Autodesk Inventor part; units mm, degrees
ref_plane "YZ Plane" through (0, 0, 0) normal (1, 0, 0) x (0, 1, 0)
ref_plane "XZ Plane" through (0, 0, 0) normal (0, 1, 0) x (-1, 0, 0)
ref_plane "XY Plane" through (0, 0, 0) normal (0, 0, 1) x (1, 0, 0)
sketch "Sketch1" plane through (0, 0, 0) normal (0, 1, 0) x (-1, 0, 0)
  line L0 (-414.3, 17.5) -> (-414.3, 107.5) construction
  line L1 (-417.5, -14.3) -> (417.5, -14.3) construction
  line L2 (417.5, 139.3) -> (-417.5, 139.3) construction
  line L3 (414.3, 107.5) -> (414.3, 17.5) construction
  line L4 (417.5, 110.7) -> (-417.5, 110.7) construction
  circle A0 centre (-400, 0) radius 2 construction
  circle A1 centre (-400, 125) radius 2 construction
  circle A2 centre (400, 0) radius 2 construction
  circle A3 centre (400, 125) radius 2 construction
  circle A4 centre (0, 125) radius 2 construction
  circle A5 centre (0, 0) radius 2 construction
  arc A6 (-255.8176, 91.7662) -> (-287.0162, 60.5676) centre (-251.75, 56.5) ccw construction
  arc A7 (-247.75, 95.5) -> (-255.75, 95.5) centre (-251.75, 95.5) ccw construction
  arc A8 (255.75, 95.5) -> (247.75, 95.5) centre (251.75, 95.5) ccw construction
  line L5 (417.5, 14.3) -> (-417.5, 14.3) construction
  line L6 (0, -14.3) -> (0, 139.3) construction
  line L7 (-414.3, 139.3) -> (414.3, 139.3)
  line L8 (414.3, 139.3) -> (414.3, -14.3)
  line L9 (-414.3, -14.3) -> (-414.3, 139.3)
  line L10 (-414.3, 139.3) -> (414.3, -14.3) construction
  line L11 (414.3, 139.3) -> (-414.3, -14.3) construction
  line L12 (-251.75, 99.5) -> (-251.75, 14.3) construction
  line L13 (251.75, 99.5) -> (251.75, 14.3) construction
  line L14 (-294.75, 56.5) -> (-294.75, -14.3)
  line L15 (-208.75, 56.5) -> (-208.75, -14.3)
  line L16 (209.15, 56.9) -> (209.15, -14.3)
  line L17 (294.35, 56.9) -> (294.35, -14.3)
  arc A9 (-260.011, 14.301) -> (-260.0059, 14.3) centre (-251.75, 56.5) ccw
  arc A10 (-208.75, 56.5) -> (-294.75, 56.5) centre (-251.75, 56.5) ccw
  arc A11 (294.35, 56.9) -> (209.15, 56.9) centre (251.75, 56.9) ccw
  line L18 (-294.75, -14.3) -> (-414.3, -14.3)
  line L19 (414.3, -14.3) -> (294.35, -14.3)
  line L20 (209.15, -14.3) -> (-208.75, -14.3)
  circle A12 centre (-400, 0) radius 3
  circle A13 centre (-400, 125) radius 3
  circle A14 centre (0, 0) radius 3
  circle A15 centre (0, 125) radius 3
  circle A16 centre (400, 125) radius 3
  circle A17 centre (400, 0) radius 3
  point P0 (0, 0)
  point P1 (0, 62.5)
  dimension "d0" = 828.6
  dimension "d1" = 43
  dimension "d2" = 125
  dimension "d3" = 1
  dimension "d4" = 1
  dimension "d5" = 1
  dimension "d6" = 1
  dimension "d7" = 1
  dimension "d8" = 1
extrude "Extrusion1" add sketch "Sketch1" along normal mid plane 2
fillet "Fillet1" radius 2 8 edges at (414.3, 0, -14.3) (208.75, 0, -14.3) (294.75, 0, -14.3) (-209.15, 0, -14.3) (-294.35, 0, -14.3) (-414.3, 0, -14.3) (414.3, 0, 139.3) (-414.3, 0, 139.3)
properties part number "Cover_LeftRight" material "Steel, Galvanized"
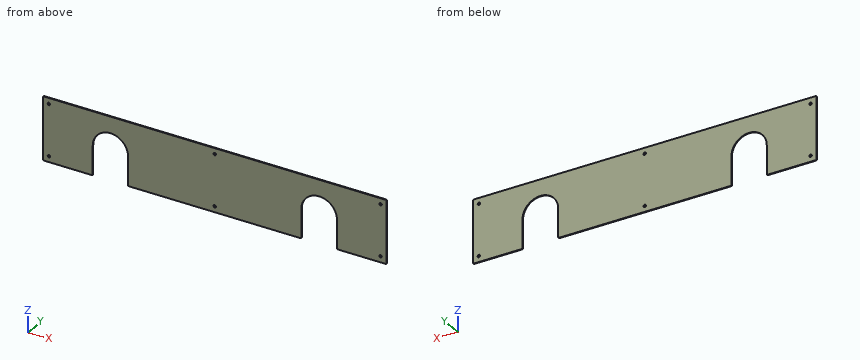
Read the model definition and answer for the solid it produces. Units are mm, in the model's axes. Coordinates: 2 decimals unless noted, no trailing zeros. Write each loop counter-clockwise with the first axis right and the second up, starting at its lowest first coordinate (ties: lowest second). Pieces come first, ordered by that corner, then holes. Notation, with made-up numbers: M 61,68.25 L 94,68.25 A12 ccw 94,81.25 Z; hole C 30,28 d5. An arc over 180 degrees is marked long. Use a Markdown table: item, result.
Q1. The part is cut by section D-D, the plane z = 81. Write down the section's boundary in (x, y).
Answer block:
| item | result |
|---|---|
| outline | M -414.3,-1 L -286.88,-1 L -286.88,1 L -414.3,1 Z; M -216.62,-1 L 216.41,-1 L 216.41,1 L -216.62,1 Z; M 287.09,-1 L 414.3,-1 L 414.3,1 L 287.09,1 Z |
Q2. The part is cut by section A-A, the plane z = 38. Write down the section's boundary in (x, y), then the cut area to 3 significant figures.
Answer block:
| item | result |
|---|---|
| outline | M -414.3,-1 L -294.35,-1 L -294.35,1 L -414.3,1 Z; M -209.15,-1 L 208.75,-1 L 208.75,1 L -209.15,1 Z; M 294.75,-1 L 414.3,-1 L 414.3,1 L 294.75,1 Z |
| area | 1,310 mm2 |
Q3. The part is cut by section B-B, the plane y = 0.7. Write down the section's boundary in (x, z).
Answer block:
| item | result |
|---|---|
| outline | M -414.3,-12.3 A2 ccw -412.3,-14.3 L -296.35,-14.3 A2 ccw -294.35,-12.3 L -294.35,56.9 A42.6 cw -209.15,56.9 L -209.15,-12.3 A2 ccw -207.15,-14.3 L 206.75,-14.3 A2 ccw 208.75,-12.3 L 208.75,56.5 A43 cw 294.75,56.5 L 294.75,-12.3 A2 ccw 296.75,-14.3 L 412.3,-14.3 A2 ccw 414.3,-12.3 L 414.3,137.3 A2 ccw 412.3,139.3 L -412.3,139.3 A2 ccw -414.3,137.3 Z; hole C -400,0 d6; hole C -400,125 d6; hole C 0,0 d6; hole C 0,125 d6; hole C 400,0 d6; hole C 400,125 d6 |
Q4. The part is cut by section C-C, the plane x = 251.75. Write down the section's boundary in (y, z), then the cut area to 3 significant figures.
Answer block:
| item | result |
|---|---|
| outline | M -1,99.5 L 1,99.5 L 1,139.3 L -1,139.3 Z |
| area | 79.6 mm2 |
Q5. Straight lines are drawn through the part: L1, parallel to Z at x = 400, y = -0.6; L2, parallel to X at y = 0.35, z = 51. For each, find the intervals that lie inside material, in ascending order. Write a range as [from, to].
Answer block:
| item | result |
|---|---|
| L1 | z = [-14.3, -3], [3, 122], [128, 139.3] |
| L2 | x = [-414.3, -294.35], [-209.15, 208.75], [294.75, 414.3] |
